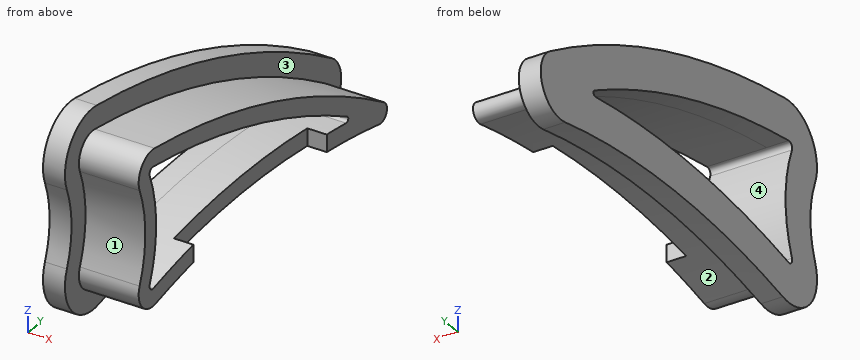
```python
from build123d import *

# Parameters (mm, degrees)
BOSS_EXTRUDE1_DEPTH = 76.2
SKETCH2_W           = 6.985
SKETCH2_H           = 9.525
CUT_EXTRUDE1_DEPTH  = 119.84173867
CUT_EXTRUDE2_DEPTH  = 119.84173867
CUT_EXTRUDE3_DEPTH  = 119.84173867
CUT_EXTRUDE4_DEPTH  = 5.08
CUT_EXTRUDE6_DEPTH  = 36.83
FILLET2_R           = 0.762
BOSS_EXTRUDE2_DEPTH = 15.5575
FILLET3_R           = 0.762
BOSS_EXTRUDE3_DEPTH = 5.715
CUT_EXTRUDE7_START  = 5.08
CUT_EXTRUDE7_DEPTH  = 5.08


with BuildPart() as part:
    # Sketch1 → Boss-Extrude1 (new body)
    with BuildSketch(Plane.XY):
        Polygon((-15.5575, 76.2), (15.5575, 76.2), (15.5575, -76.2), (7.845485509, -76.2), (9.525, -85.725), (-9.525, -85.725), (-7.845485509, -76.2), (-15.5575, -76.2), align=None)
    extrude(amount=BOSS_EXTRUDE1_DEPTH)

    # Sketch2 → Cut-Extrude1 (cut, through all)
    with BuildSketch(Plane(origin=(15.5575, 0, 0), x_dir=(0, 0, -1), z_dir=(1, 0, 0))):
        with Locations((-3.4925, -80.9625)):
            Rectangle(SKETCH2_W, SKETCH2_H)
    extrude(amount=-CUT_EXTRUDE1_DEPTH, mode=Mode.SUBTRACT)

    # Sketch3 → Cut-Extrude2 (cut, through all)
    with BuildSketch(Plane(origin=(15.5575, 0, 0), x_dir=(0, 0, -1), z_dir=(1, 0, 0))):
        with BuildLine():
            Line((-76.2, -85.725), (-76.2, -76.2))
            Line((-76.2, -76.2), (-76.2, 76.2))
            Line((-76.2, 76.2), (-15.907508532, 76.2))
            ThreePointArc((-15.907508532, 76.2), (-60.637785123, 0.667838465), (-76.2, -85.725))
        make_face()
        with BuildLine():
            Line((0, -76.2), (0, 63.796446855))
            ThreePointArc((0, 63.796446855), (-12.85182234, -6.201776572), (0, -76.2))
        make_face()
    extrude(amount=-CUT_EXTRUDE2_DEPTH, mode=Mode.SUBTRACT)

    # Sketch6 → Cut-Extrude3 (cut, through all)
    with BuildSketch(Plane(origin=(15.5575, 0, 0), x_dir=(0, 0, -1), z_dir=(1, 0, 0))):
        with BuildLine():
            ThreePointArc((-26.004408293, 40.411420838), (-22.895186728, 41.391641282), (-21.382101704, 38.503966686))
            ThreePointArc((-21.382101704, 38.503966686), (-26.183938112, -7.303408092), (-20.902654077, -53.057984431))
            ThreePointArc((-20.902654077, -53.057984431), (-22.751384732, -58.666992363), (-28.575599954, -59.645405394))
            ThreePointArc((-28.575599954, -59.645405394), (-40.728748793, -57.329846812), (-52.881897632, -59.645405394))
            ThreePointArc((-52.881897632, -59.645405394), (-58.514495406, -58.82440967), (-60.644203683, -53.545722871))
            ThreePointArc((-60.644203683, -53.545722871), (-48.403726567, -4.694487773), (-26.004408293, 40.411420838))
        make_face()
    extrude(amount=-CUT_EXTRUDE3_DEPTH, mode=Mode.SUBTRACT)

    # Sketch7 → Cut-Extrude4 (cut, symmetric)
    with BuildSketch(Plane(origin=(0, 0, 0), x_dir=(0, 0, -1), z_dir=(1, 0, 0))):
        with BuildLine():
            Line((-24.910956945, 16.933040929), (-11.489033389, 16.933040929))
            ThreePointArc((-11.489033389, 16.933040929), (-12.80682615, -10.412600109), (-10.321792572, -37.676959071))
            Line((-10.321792572, -37.676959071), (-23.81904356, -37.676959071))
            ThreePointArc((-23.81904356, -37.676959071), (-26.144779891, -10.407545323), (-24.910956945, 16.933040929))
        make_face()
    extrude(amount=CUT_EXTRUDE4_DEPTH, both=True, mode=Mode.SUBTRACT)

    # Sketch10 → Cut-Extrude6 (cut, symmetric)
    with BuildSketch(Plane(origin=(15.5575, 76.2, 15.907508532), x_dir=(-1, 0, 0), z_dir=(0, -0.6148991463064188, -0.7886057569353888))):
        Polygon((0, 9.781513416), (8.255, 9.781513416), (0, -2.283486584), align=None)
        Polygon((31.115, 9.781513416), (31.115, -2.283486584), (22.86, 9.781513416), align=None)
    extrude(amount=CUT_EXTRUDE6_DEPTH, both=True, mode=Mode.SUBTRACT)

    # Fillet2
    fillet2_edges = [part.edges().sort_by_distance(p)[0] for p in [
        (0, 76.2, 15.907508532),
        (-14.77625063, 75.333628159, 16.653053168),
        (14.77625063, 75.333628159, 16.653053168),
        (-15.5575, 4.051612744, 59.349592349),
        (15.5575, 4.051612744, 59.349592349),
    ]]
    fillet(fillet2_edges, radius=FILLET2_R)


with BuildPart() as body_2:
    # Sketch11 → Boss-Extrude2 (new body)
    with BuildSketch(Plane(origin=(15.5575, 0, 0), x_dir=(0, 0, -1), z_dir=(1, 0, 0))):
        with BuildLine():
            ThreePointArc((-60.644203683, -53.545722871), (-58.514495406, -58.82440967), (-52.881897632, -59.645405394))
            ThreePointArc((-52.881897632, -59.645405394), (-40.728748793, -57.329846812), (-28.575599954, -59.645405394))
            ThreePointArc((-28.575599954, -59.645405394), (-22.751384732, -58.666992363), (-20.902654077, -53.057984431))
            ThreePointArc((-20.902654077, -53.057984431), (-26.183938112, -7.303408092), (-21.382101704, 38.503966686))
            ThreePointArc((-21.382101704, 38.503966686), (-22.895186728, 41.391641282), (-26.004408293, 40.411420838))
            ThreePointArc((-26.004408293, 40.411420838), (-48.403726567, -4.694487773), (-60.644203683, -53.545722871))
        make_face()
        with BuildLine():
            ThreePointArc((-56.241344514, -54.156342338), (-55.768076008, -55.329383849), (-54.516387613, -55.511827344))
            ThreePointArc((-54.516387613, -55.511827344), (-40.728748793, -52.884846812), (-26.941109972, -55.511827344))
            ThreePointArc((-26.941109972, -55.511827344), (-25.646839923, -55.294402226), (-25.236010888, -54.047956018))
            ThreePointArc((-25.236010888, -54.047956018), (-30.535382276, -12.638178349), (-27.725713329, 29.014658098))
            ThreePointArc((-27.725713329, 29.014658098), (-45.998284717, -11.194361196), (-56.241344514, -54.156342338))
        make_face(mode=Mode.SUBTRACT)
    extrude(amount=-BOSS_EXTRUDE2_DEPTH)

    # Fillet3
    fillet3_edges = [body_2.edges().sort_by_distance(p)[0] for p in [
        (7.77875, 29.014658098, 27.725713329),
    ]]
    fillet(fillet3_edges, radius=FILLET3_R)

    # Sketch13 → Cut-Extrude7 (cut)
    with BuildSketch(Plane(origin=(0, 0, 0), x_dir=(0, 0, -1), z_dir=(1, 0, 0)).offset(CUT_EXTRUDE7_START)):
        with BuildLine():
            Line((-11.489033389, 16.933040929), (-29.382511575, 16.933040929))
            ThreePointArc((-29.382511575, 16.933040929), (-30.590678841, -10.406069442), (-28.313574796, -37.676959071))
            Line((-28.313574796, -37.676959071), (-10.321792572, -37.676959071))
            ThreePointArc((-10.321792572, -37.676959071), (-12.80682615, -10.412600109), (-11.489033389, 16.933040929))
        make_face()
    extrude(amount=-CUT_EXTRUDE7_DEPTH, mode=Mode.SUBTRACT)


with BuildPart() as body_3:
    # Sketch12 → Boss-Extrude3 (new body)
    with BuildSketch(Plane(origin=(15.5575, 0, 0), x_dir=(0, 0, -1), z_dir=(1, 0, 0))):
        with BuildLine():
            ThreePointArc((-30.820115457, 43.488788141), (-53.765912925, -2.717575417), (-66.305022615, -52.760640699))
            ThreePointArc((-66.305022615, -52.760640699), (-62.045606061, -63.318014297), (-50.780410512, -64.960005745))
            ThreePointArc((-50.780410512, -64.960005745), (-40.728748793, -63.044846812), (-30.677087073, -64.960005745))
            ThreePointArc((-30.677087073, -64.960005745), (-19.028656629, -63.003179683), (-15.331195319, -51.785163819))
            ThreePointArc((-15.331195319, -51.785163819), (-20.469016461, -7.273482937), (-15.797619041, 37.289562147))
            ThreePointArc((-15.797619041, 37.289562147), (-20.715145369, 46.674504585), (-30.820115457, 43.488788141))
        make_face()
        with BuildLine():
            ThreePointArc((-56.241344514, -54.156342338), (-55.768076008, -55.329383849), (-54.516387613, -55.511827344))
            ThreePointArc((-54.516387613, -55.511827344), (-40.728748793, -52.884846812), (-26.941109972, -55.511827344))
            ThreePointArc((-26.941109972, -55.511827344), (-25.646839923, -55.294402226), (-25.236010888, -54.047956018))
            ThreePointArc((-25.236010888, -54.047956018), (-30.462301973, -14.734514328), (-28.372972672, 24.869721798))
            ThreePointArc((-28.372972672, 24.869721798), (-28.883789244, 25.702089435), (-29.794040566, 25.34823638))
            ThreePointArc((-29.794040566, 25.34823638), (-46.671799333, -13.18850949), (-56.241344514, -54.156342338))
        make_face(mode=Mode.SUBTRACT)
    extrude(amount=BOSS_EXTRUDE3_DEPTH)


with BuildPart() as body_2_1:
    add(body_2.part)

    # Combine1: union body 3
    add(body_3.part)


with BuildPart() as body_2_2:
    # Mirror1: mirrored copy
    add(body_2_1.part.mirror(Plane(origin=(0, -70.027902522, -58.200215313), x_dir=(0, 0, 1), z_dir=(1, 0, 0))))


solid = body_2_2.part
```
Part model, mm, in its own coordinate system. Face numbers are marked on the shaded views. A direction names the side the tool comes from. Round coordinates to 2 decimals unless told otherwise and drop trailing zeros. Write each loop counter-clockwise with the first axis right and the second up, starting at its lowest first coordinate (ties: lowest second). Pieces come first, ordered by that corner, then holes. Notation, with made-up numbers: (18.5, -27) -> (52.5, -27) arc R35 ccw to (52.5, 7) -> close; hole circle Ø2 at (-23.75, -9). An arc over 180 degrees is marked (long way). Return JSON: item names as keys, results as strings. Group by question number.
Q1. Saw through at D-D on z = 35.5. Write the cut outline in (x, y), plus the area to 3 significant figures.
Q2. Saw through at B-B on z = 18. Write the cut outline in (x, y).
Q3. Pin check, flat tips, straight feed: pin 1 (6 mm diameter, centred on x = -8.5, y = -43, fed in from -Z); pin 2 (10 mm diameter, centred on x = -13.5, y = -4, fed in from -Z); pin 3 (1.3 mm diameter, centred on x = -3.5, z = 25.5, fed in from +Y). Stop position of each tip, or through.
Q4. Saw through at A-A on y = -20. Write the cut outline in (x, z).
Q5. Probe L1, parallel to X at y = 33.5, z = 33; L2, parallel to Y at x = -9, z = 31; L3, parallel to Z at x = -15, y = -8. List the from-to ranges inside material, lowest first. Write a range as [from, to].
Q6. Saw through at C-C on y = -46.5. Write the cut outline in (x, z).
Q7. Which spindle directions (+Z, -Z, +X, -X, +Y, -Y) get a long thin tool onto all of the face, cutting with end or side? Do the marked faces 1, 2, 3 and 4. Say none if no direction does.
Answer:
{
 "1": {"outline": "(-21.27, -63.55) -> (-15.56, -63.55) -> (-15.56, -57.75) -> (0, -57.75) -> (0, -53.25) -> (-21.27, -53.25) -> close; (-21.27, 14.32) -> (0, 14.32) -> (0, 24.15) -> (-15.56, 24.15) -> (-15.56, 35.86) -> (-21.27, 35.86) -> close", "area": "405 mm2"},
 "2": {"outline": "(-21.27, -62) -> (-15.56, -62) -> (-15.56, -37.91) -> (-21.27, -37.91) -> close; (-21.27, 25.51) -> (-15.56, 25.51) -> (-15.56, 44.85) -> (-21.27, 44.85) -> close"},
 "3": {"pin 1": "z = 22.39", "pin 2": "z = 20.36", "pin 3": "y = 41.38"},
 "4": {"outline": "(-21.27, 20.01) -> (-15.56, 20.01) -> (-15.56, 25.73) -> (-5.08, 25.73) -> (-5.08, 30.19) -> (-21.27, 30.19) -> close; (-21.27, 48.82) -> (0, 48.82) -> (0, 53.46) -> (-15.56, 53.46) -> (-15.56, 59.4) -> (-21.27, 59.4) -> close"},
 "5": {"L1": "[-21.27, -15.56]", "L2": "[-58.79, -54.17], [23.14, 32.23]", "L3": "[26.18, 30.62], [44.88, 49.59]"},
 "6": {"outline": "(-21.27, 16.47) -> (-15.56, 16.47) -> (-15.56, 22.29) -> (0, 22.29) -> (0, 26.82) -> (-21.27, 26.82) -> close; (-21.27, 55.05) -> (0, 55.05) -> (0, 59.56) -> (-15.56, 59.56) -> (-15.56, 65.35) -> (-21.27, 65.35) -> close"},
 "7": {"face 1": "+X, -Y", "face 2": "-Z, +X", "face 3": "+X", "face 4": "+X, -X"}
}
